Autodesk Inventor part; units mm, degrees
ref_plane "YZ Plane" through (0, 0, 0) normal (1, 0, 0) x (0, 1, 0)
ref_plane "XZ Plane" through (0, 0, 0) normal (0, 1, 0) x (-1, 0, 0)
ref_plane "XY Plane" through (0, 0, 0) normal (0, 0, 1) x (1, 0, 0)
sketch "Sketch1" plane through (0, 0, 0) normal (0, 0, 1) x (1, 0, 0)
  circle A0 centre (0, 0) radius 5 construction
  circle A1 centre (0, 0) radius 5.05
  line L0 (-11, 12.5) -> (11, 12.5)
  line L1 (11, 12.5) -> (11, -52.3463)
  line L2 (11, -52.3463) -> (-11, -52.3463)
  line L3 (-11, -52.3463) -> (-11, 12.5)
  circle A2 centre (0, 0) radius 12.5 construction
  circle A3 centre (4.5, -18.5109) radius 6.5 construction
  circle A4 centre (4.5, -18.5109) radius 7.5 construction
  circle A5 centre (4.5, -18.5109) radius 4
  circle A6 centre (24.9354, -38.9463) radius 21.4 construction
  line L4 (4.5, -18.5109) -> (24.9354, -38.9463) construction
  line L5 (0, 48.1253) -> (0, -78.4249) construction
  circle A7 centre (0, 0) radius 19.05 construction
  line L6 (54.9772, -60.3463) -> (-51.313, -60.3463) construction
  line L7 (-70.5727, -54.3463) -> (77.7123, -54.3463) construction
  line L8 (8, -57.4182) -> (8, 30.0467) construction
  circle A8 centre (8, -36.8463) radius 1.5
  circle A9 centre (0, 0) radius 11 construction
  line L9 (12, -6.3386) -> (12, -55.2043) construction
  dimension "d8" = 38.1
  dimension "d0" = 10
  dimension "d1" = 10.1
  dimension "d2" = 25
  dimension "d3" = 13
  dimension "d4" = 15
  dimension "d5" = 8
  dimension "d6" = 42.8
  dimension "d7" = 45
  dimension "d9" = 6
  dimension "d10" = 2
  dimension "d11" = 3
  dimension "d12" = 3
  dimension "d27" = 22
  dimension "d71" = 15.5
  dimension "d84" = 64.8463
  dimension "d85" = 1
extrude "Extrusion1" add sketch "Sketch1" along normal blind 3
sketch "Sketch2" plane through (0, 0, 0) normal (0, 0, -1) x (-1, 0, 0)
  circle A0 centre (0, 0) radius 8.5 construction
  line L0 (-15.4, 0) -> (15.4, 0) construction
  point P0 (-8.5, 0)
  point P1 (-4.25, -7.3612)
  point P2 (4.25, -7.3612)
  point P3 (8.5, 0)
  point P4 (4.25, 7.3612)
  point P5 (-4.25, 7.3612)
  dimension "d15" = 17
  dimension "d18" = 360
hole "Hole1" at (8.5, 0, 0) at (4.25, -7.3612, 0) at (-4.25, -7.3612, 0) at (-8.5, 0, 0) at (-4.25, 7.3612, 0) at (4.25, 7.3612, 0) direction (0, 0, 1) diameter 2 end through all counterbore diameter 4 counterbore depth 2
sketch "Sketch3" plane through (0, 0, 3) normal (0, 0, 1) x (1, 0, 0)
  circle A0 centre (-3, -29.6963) radius 6.05 construction
  circle A1 centre (-3, -44.2963) radius 6.05 construction
  line L0 (-3, -52.9991) -> (-3, -16.007) construction
  line L1 (0, 25.5998) -> (0, -66.099) construction
  line L2 (-19.4661, -50.3463) -> (34.3963, -50.3463) construction
  line L3 (-11, -52.3463) -> (11, -52.3463) construction
  line L4 (-9.05, -29.6963) -> (-9.05, -44.2963)
  line L5 (3.05, -29.6963) -> (3.05, -44.2963)
  arc A2 (3.05, -29.6963) -> (-9.05, -29.6963) centre (-3, -29.6963) ccw
  arc A3 (-9.05, -44.2963) -> (3.05, -44.2963) centre (-3, -44.2963) ccw
  point P0 (0, 0)
  dimension "d28" = 12.1
  dimension "d29" = 14.6
  dimension "d30" = 3
  dimension "d31" = 2
extrude "Extrusion2" cut sketch "Sketch3" against normal through all
sketch "Sketch4" plane through (0, 0, 3) normal (0, 0, 1) x (1, 0, 0)
  circle A0 centre (0, 0) radius 13 construction
  circle A1 centre (4.5, -18.5109) radius 4 construction
  circle A2 centre (4.5, -18.5109) radius 7 construction
  line L0 (-30.9627, -14.5) -> (22.7085, -14.5) construction
  line L1 (-11, 12.5) -> (-11, -52.3463) construction
  line L2 (11, 12.5) -> (-11, 12.5) construction
  line L3 (-11, -12.7679) -> (-8, -11.0359) construction
  line L4 (-8, -11.0359) -> (-5, -12.7679) construction
  line L5 (-5, -12.7679) -> (-5, -16.2321) construction
  line L6 (-5, -16.2321) -> (-8, -17.9641) construction
  line L7 (-8, -17.9641) -> (-11, -16.2321) construction
  line L8 (-11, -16.2321) -> (-11, -12.7679) construction
  circle A3 centre (-8, -14.5) radius 2.8 construction
  dimension "d34" = 26
  dimension "d35" = 14
  dimension "d36" = 6
  dimension "d37" = 27
  dimension "d72" = 5.6
hole "Hole2" at (-8, -14.5, 3) direction (0, 0, -1) diameter 3 end through all
ref_plane "Work Plane1" through (-3, -29.6963, 3) normal (-1, 0, 0) x (0, 0, -1)
sketch "Sketch8" plane through (0, 0, 3) normal (0, 0, 1) x (1, 0, 0)
  line L0 (11, 12.5) -> (-11, 12.5)
  line L1 (-11, 12.5) -> (-19, 12.5)
  line L2 (-19, 12.5) -> (-19, 4.5)
  line L3 (-19, 4.5) -> (-11, 4.5)
  line L4 (-11, 4.5) -> (-11, 12.5)
  point P0 (0, 0)
  dimension "d58" = 8
  dimension "d59" = 8
extrude "Extrusion4" add sketch "Sketch8" against normal up to surface (3 mm away)
sketch "Sketch9" plane through (0, 0, 3) normal (0, 0, 1) x (1, 0, 0)
  line L0 (-19, 12.5) -> (-19, 4.5) construction
  line L1 (-19, 8.5) -> (-9.7013, 8.5) construction
  line L2 (11, 12.5) -> (-19, 12.5) construction
  line L3 (-16, 12.5) -> (-16, 1.2197) construction
  point P0 (0, 0)
  point P1 (-16, 8.5)
  dimension "d62" = 3
hole "Hole4" at (-16, 8.5, 3) direction (0, 0, -1) diameter 3 end through all
fillet "Fillet2" radius 2 6 edges at (11, -52.3463, 1.5) (-11, -52.3463, 1.5) (11, 12.5, 1.5) (-19, 12.5, 1.5) (-19, 4.5, 1.5) (-11, 4.5, 1.5)
sketch "Sketch12" plane through (0, 0, 3) normal (0, 0, 1) x (1, 0, 0)
  circle A0 centre (8, -36.8463) radius 1.5 construction
  line L0 (8, -27.4514) -> (8, -47.8605) construction
  line L1 (24.4744, -26.8463) -> (0, -26.8463) construction
  line L2 (-0.5807, -45.3463) -> (23.4788, -45.3463) construction
  line L3 (0.6637, -29.8463) -> (21.6536, -29.8463) construction
  line L4 (0, -42.3463) -> (23.4788, -42.3463) construction
  point P0 (0, 0)
  point P1 (8, -29.8463)
  point P2 (8, -42.3463)
  dimension "d73" = 10
  dimension "d74" = 8.5
  dimension "d75" = 3
  dimension "d76" = 3
hole "Hole5" at (8, -29.8463, 3) at (8, -42.3463, 3) direction (0, 0, -1) diameter 2.013 end through all
sketch "Sketch13" plane through (0, 0, 3) normal (0, 0, 1) x (1, 0, 0)
  line L0 (-19, 10.5) -> (-19, 6.5) construction
  line L1 (9, 12.5) -> (-17, 12.5) construction
  line L2 (-19, 10.5) -> (-19, 15.5)
  line L3 (-19, 15.5) -> (-11, 15.5)
  line L4 (-11, 15.5) -> (-11, 12.5)
  line L5 (-11, 2.5) -> (-11, -50.3463)
  arc A0 (-17, 12.5) -> (-19, 10.5) centre (-17, 10.5) ccw
  line L6 (-17, 12.5) -> (-11, 12.5)
  point P0 (0, 0)
  dimension "d86" = 3
extrude "Extrusion5" add sketch "Sketch13" against normal up to surface (3 mm away)
fillet "Fillet3" radius 2 3 edges at (-19, 15.5, 1.5) (-11, 15.5, 1.5) (-11, 12.5, 1.5)
equation "\"d8\" = d2 + d3 + tol"
equation "\"d4\" = roller_diam"
equation "\"d5\" = roller_bearing_dia"
equation "\"d7\" = ball_roller_angle"
equation "\"d28\" = absorber_dia"
equation "\"d29\" = absorber_dia + absorber_length"
equation "\"tol\" = 0.1"
equation "\"z_motor\" = 50"
equation "\"z_roller\" = 26"
equation "\"pitch\" = 0.5"
equation "\"roller_diam\" = 15"
equation "\"roller_bearing_dia\" = 8"
equation "\"ball_roller_angle\" = 45deg"
equation "\"absorber_dia\" = 12.1"
equation "\"absorber_length\" = 2.5"
properties part number "side_plate" material "Aluminum 6061"
CAD build for the part. Positions are in the model's coordinates, mm. A direction names the side the tool comes from. Coordinates: 2 decimals unless noted, no trailing zeros. Order: outer loops, then holes, each group sorted by start corner. A loop starts at its lowest first (then second) coordinate and runs counter-clockwise, first axis right, second up. Notation, with made-up numbers: (3, 54) - (31, 54) arc R20 cw to (31, 64) - close; hole circle Ø4 at (32, -4.5). An arc over 180 degrees is marked (long way). Answer in a Markdown table with one row per item.
1. Slice it at B-B, the plane x = -16. List the corners of the cut face in (y, z).
Answer:
| item | result |
|---|---|
| outline | (4.5, 0) - (7, 0) - (7, 3) - (4.5, 3) - close; (10, 0) - (15.5, 0) - (15.5, 3) - (10, 3) - close |
2. Slice it at A-A, the plane y = 0. List the corners of the cut face in (x, z), then the cut area to 3 significant figures.
Answer:
| item | result |
|---|---|
| outline | (-11, 0) - (-10.5, 0) - (-10.5, 2) - (-9.5, 2) - (-9.5, 3) - (-11, 3) - close; (-7.5, 2) - (-6.5, 2) - (-6.5, 0) - (-5.05, 0) - (-5.05, 3) - (-7.5, 3) - close; (5.05, 0) - (6.5, 0) - (6.5, 2) - (7.5, 2) - (7.5, 3) - (5.05, 3) - close; (9.5, 2) - (10.5, 2) - (10.5, 0) - (11, 0) - (11, 3) - (9.5, 3) - close |
| area | 15.7 mm² |
3. 3-axis set-ups, long thin cutter, end or side, ignore diameter. For faces 5 (the face through (-3.133, -50.345, 1.521)), 6 (the face through (0, -52.346, 1)), 7 (the face through (-10.43, -51.745, 1.521)), 8 (the face through (-3.484, -5.514, 1.014)), 9 (the face through (0, 12.5, 2)): which of +Z, -Z, +X, -X, +Y, -Y reach the whole face in a straight line?
Answer:
| item | result |
|---|---|
| face 5 | +Z, -Z |
| face 6 | +Z, -Z, +X, -X, -Y |
| face 7 | +Z, -Z, -X, -Y |
| face 8 | -Z |
| face 9 | +Z, -Z, +X, +Y |
4. Slice it at C-C, the plane y = -40. List the corners of the cut face in (x, z).
Answer:
| item | result |
|---|---|
| outline | (-11, 0) - (-9.05, 0) - (-9.05, 3) - (-11, 3) - close; (3.05, 0) - (11, 0) - (11, 3) - (3.05, 3) - close |
5. Flat gauge pins, fed straight in: P1, Ø3, axis at x = 8.5, y = 0, coming from the +Z side; P2, Ø1.2, axis at x = 9, y = 0.5, coming from the -Z side; P3, Ø1.5, axis at x = -5, z = 2, coming from the +Y side. Where does each tip first touch, or does it go through?
Answer:
| item | result |
|---|---|
| P1 | z = 3 |
| P2 | z = 2 |
| P3 | y = 12.5 |
6. Slice it at D-D, the plane x = -1.5. List the corners of the cut face in (y, z), then the cut area to 3 significant figures.
Answer:
| item | result |
|---|---|
| outline | (-52.35, 0) - (-50.16, 0) - (-50.16, 3) - (-52.35, 3) - close; (-23.84, 0) - (-4.82, 0) - (-4.82, 3) - (-23.84, 3) - close; (4.82, 0) - (12.5, 0) - (12.5, 3) - (4.82, 3) - close |
| area | 86.6 mm² |
7. Pull direction Y, two halves, no side cores. Call faces 1 (the face through (6.517, -0.26, 1.014)), 2 (the face through (-18.43, 14.9, 1.48)), 3 (the face through (-15, 4.5, 2)), 4 (the face through (11, -19, 1)): +Y half, -Y half, draft (parallel to the pull), parting line (faces both ways), or undercut.
Answer:
| item | result |
|---|---|
| face 1 | undercut |
| face 2 | +Y half |
| face 3 | -Y half |
| face 4 | draft |
8. Drill centre lines: L1, parallel to X at y = -42.5, z = 1.75; L2, parallel to X at y = -41.5, z = 2.2; L3, parallel to Y at x = -4.25, z = 2.65. Where is each one in solid material? Low to high. Write a range as from..to.
Answer:
| item | result |
|---|---|
| L1 | -11..-9.05, 3.05..7.01, 8.99..11 |
| L2 | -11..-9.05, 3.05..7.46, 8.54..11 |
| L3 | -52.35..-50.22, -23.78..-8.36, -6.36..-2.73, 2.73..6.36, 8.36..12.5 |
